The figure shows three views and two pictorial views of one solid part (mm, origin at its lowest corner). Answer the questions. Round coordinates to 2 decimals unless told otherwise and drop trailing zeros. Order: outer loops, then holes, each group sorted by start corner. A loop starts at its lowest first (then second) coordinate and runs counter-clockwise, first axis right, second up. Notation, with made-up numbers: M -20,-6 L -4,-6 A26 cw -4,24 Z; hole C 86.5,-18.5 d6. An arc over 180 degrees is marked long. Return JSON: item names as keys, results as strings.
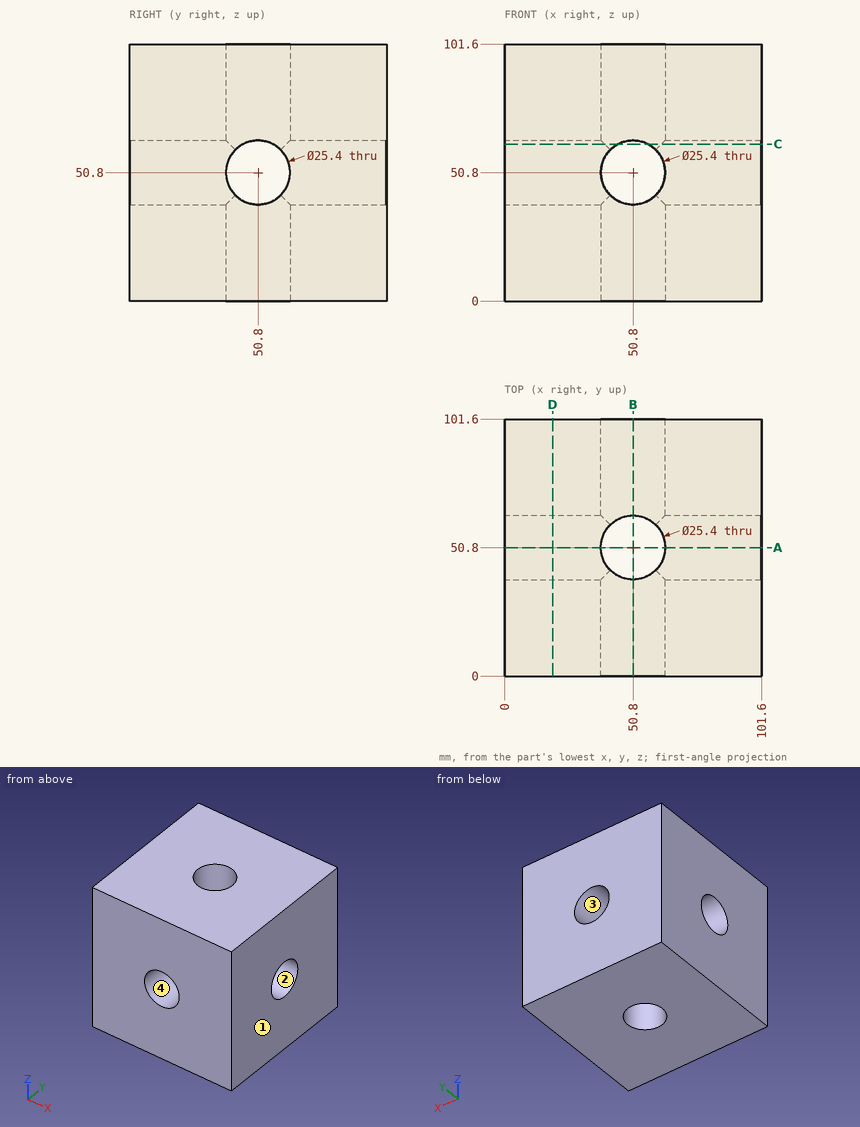
Item 1: Find section C-C (z = 62). Determine the outline of the cut face in (x, y), plus the area to 3 significant figures.
Output:
{"outline": "M 0,0 L 44.81,0 L 44.81,39.6 A12.7 cw 39.6,44.81 L 0,44.81 Z; M 0,56.79 L 39.6,56.79 A12.7 cw 44.81,62 L 44.81,101.6 L 0,101.6 Z; M 56.79,0 L 101.6,0 L 101.6,44.81 L 62,44.81 A12.7 cw 56.79,39.6 Z; M 56.79,62 A12.7 cw 62,56.79 L 101.6,56.79 L 101.6,101.6 L 56.79,101.6 Z", "area": "7,970 mm^2"}
Item 2: The mould has two halves that part along X. Classify the marked faces 1, 2, 3 and 4: pulls with the +X half, pulls with the -X half, needs draft (parallel to the pull), parting line crosses it, or undercut.
Output:
{"face 1": "pulls with the +X half", "face 2": "needs draft", "face 3": "undercut", "face 4": "undercut"}
Item 3: Find section D-D (x = 19). Determine the outline of the cut face in (y, z), plus the area to 3 significant figures.
Output:
{"outline": "M 0,0 L 101.6,0 L 101.6,101.6 L 0,101.6 Z; hole C 50.8,50.8 d25.4", "area": "9,820 mm^2"}
Item 4: Find section A-A (y = 50.8). Determine the outline of the cut face in (x, z), plus the area to 3 significant figures.
Output:
{"outline": "M 0,0 L 38.1,0 L 38.1,38.1 L 0,38.1 Z; M 0,63.5 L 38.1,63.5 L 38.1,101.6 L 0,101.6 Z; M 63.5,0 L 101.6,0 L 101.6,38.1 L 63.5,38.1 Z; M 63.5,63.5 L 101.6,63.5 L 101.6,101.6 L 63.5,101.6 Z", "area": "5,810 mm^2"}
Item 5: This flat-tipped pin is pushed along its axis until it touches: pin 1 (1.5 mm diameter, centred on x = 53.5, y = 39, fed in from +Z). Where does it stop, or does it pass through?
Output:
{"pin 1": "stops at z = 101.6"}
Item 6: Consider line 1 along X through (y, z) = (50.8, 85.5); line 2 along Y through (x, z) = (9, 40). Determine where each line is inside the solid, lowest interval first. Write a range as [from, to].
Output:
{"line 1": "x = [0, 38.1], [63.5, 101.6]", "line 2": "y = [0, 44.12], [57.48, 101.6]"}
